from build123d import *

# Parameters (mm, degrees)
BOSS_EXTRU_1_DEPTH      = 7
CONG_1_R                = 1
COQUE1_T                = -0.3
ENL_V_MAT_EXTRU_1_REACH = 9
ESQUISSE8_R             = 4.427961532
ENL_V_MAT_EXTRU_2_REACH = 9
ESQUISSE9_W             = 4.325203416
ESQUISSE9_H             = 7.820915767
ENL_V_MAT_EXTRU_3_REACH = 9
ESQUISSE10_W            = 4.799198311
ESQUISSE10_H            = 8.413409385


with BuildPart() as part:
    # Esquisse3 → Boss.-Extru.1 (new body)
    with BuildSketch(Plane(origin=(0, 0, 0), x_dir=(1, 0, 0), z_dir=(0, 1, 0))):
        with BuildLine():
            Line((-26.504477612, 19.954228856), (25.695522388, 19.954228856))
            ThreePointArc((25.695522388, 19.954228856), (26.402629169, 19.661335637), (26.695522388, 18.954228856))
            Line((26.695522388, 18.954228856), (26.695522388, -23.245771144))
            ThreePointArc((26.695522388, -23.245771144), (26.402629169, -23.952877925), (25.695522388, -24.245771144))
            Line((25.695522388, -24.245771144), (-26.504477612, -24.245771144))
            ThreePointArc((-26.504477612, -24.245771144), (-27.211584393, -23.952877925), (-27.504477612, -23.245771144))
            Line((-27.504477612, -23.245771144), (-27.504477612, 18.954228856))
            ThreePointArc((-27.504477612, 18.954228856), (-27.211584393, 19.661335637), (-26.504477612, 19.954228856))
        make_face()
    extrude(amount=BOSS_EXTRU_1_DEPTH)

    # Congé1
    cong_1_edges = [part.edges().sort_by_distance(p)[0] for p in [
        (26.402629169, 7, -19.661335637),
        (26.695522388, 7, 2.145771144),
        (26.402629169, 7, 23.952877925),
        (-0.404477612, 7, 24.245771144),
        (-27.211584393, 7, 23.952877925),
        (-27.504477612, 7, 2.145771144),
        (-27.211584393, 7, -19.661335637),
        (-0.404477612, 7, -19.954228856),
    ]]
    fillet(cong_1_edges, radius=CONG_1_R)

    # Coque1
    coque1_openings = [part.faces().sort_by_distance(p)[0] for p in [
        (-0.404477612, 0, 2.145771144),
    ]]
    offset(amount=COQUE1_T, openings=coque1_openings, kind=Kind.INTERSECTION)

    # Esquisse8 → Enlèv. mat.-Extru.1 (cut, up to next)
    with BuildSketch(Plane(origin=(0, 7, 0), x_dir=(1, 0, 0), z_dir=(0, 1, 0)), mode=Mode.PRIVATE) as enl_v_mat_extru_1_sk1:
        with Locations((-4.865513773, -1.564595223)):
            Circle(ESQUISSE8_R)
    enl_v_mat_extru_1_tool1 = extrude(enl_v_mat_extru_1_sk1.sketch, amount=-ENL_V_MAT_EXTRU_1_REACH, mode=Mode.PRIVATE) & part.part
    add(enl_v_mat_extru_1_tool1.solids().sort_by_distance((-4.865514, 7, 1.564595))[0], mode=Mode.SUBTRACT)

    # Esquisse9 → Enlèv. mat.-Extru.2 (cut, up to next)
    with BuildSketch(Plane(origin=(0, 7, 0), x_dir=(1, 0, 0), z_dir=(0, 1, 0)), mode=Mode.PRIVATE) as enl_v_mat_extru_2_sk1:
        with Locations((-12.89117049, 11.513635006)):
            Rectangle(ESQUISSE9_W, ESQUISSE9_H)
    enl_v_mat_extru_2_tool1 = extrude(enl_v_mat_extru_2_sk1.sketch, amount=-ENL_V_MAT_EXTRU_2_REACH, mode=Mode.PRIVATE) & part.part
    add(enl_v_mat_extru_2_tool1.solids().sort_by_distance((-12.89117, 7, -11.513635))[0], mode=Mode.SUBTRACT)

    # Esquisse10 → Enlèv. mat.-Extru.3 (cut, up to next)
    with BuildSketch(Plane(origin=(0, 7, 0), x_dir=(1, 0, 0), z_dir=(0, 1, 0)), mode=Mode.PRIVATE) as enl_v_mat_extru_3_sk1:
        with Locations((21.532708754, -8.690397391)):
            Rectangle(ESQUISSE10_W, ESQUISSE10_H)
    enl_v_mat_extru_3_tool1 = extrude(enl_v_mat_extru_3_sk1.sketch, amount=-ENL_V_MAT_EXTRU_3_REACH, mode=Mode.PRIVATE) & part.part
    add(enl_v_mat_extru_3_tool1.solids().sort_by_distance((21.532709, 7, 8.690397))[0], mode=Mode.SUBTRACT)


solid = part.part
Read the model definition and answer for the solid it produces. Units are mm, in the model's axes. A direction names the side the tool comes from. Coordinates: 2 decimals unless noted, no trailing zeros. Write each loop counter-clockwise with the first axis right and the second up, starting at its lowest first coordinate (ties: lowest second). Pieces come first, ordered by that corner, then holes. Notation, with made-up numbers: M -24,40.5 L 28,40.5 A30 cw 28,78.5 Z; hole C -7,-2 d5. An arc over 180 degrees is marked long. Use a Markdown table: item, result.
Q1. Each of these flat-tipped pins is pushed along its axis until it touches: pin 1 Ø10 at (x, z) = (-4.87, 1.56) entering from +Y; pin 2 Ø3 at (x, z) = (20.5, -2) entering from -Y. Where does it stop, or does it pass through?
Answer block:
| item | result |
|---|---|
| pin 1 | stops at y = 7 |
| pin 2 | stops at y = 6.7 |
Q2. Straight lines are drawn through the part: L1, parallel to X at y = 0.5, z = -1; L2, parallel to Z at x = -17.5, y = 3.5; L3, parallel to Y at x = -15.5, z = 17. For each, find the intervals that lie inside material, in ascending order. Write a range as [from, to].
Answer block:
| item | result |
|---|---|
| L1 | x = [-27.5, -27.2], [26.4, 26.7] |
| L2 | z = [-19.95, -19.65], [23.95, 24.25] |
| L3 | y = [6.7, 7] |
Q3. Determine the mould class of faces 3 (the face through (-1, 3, -19.954)), 4 (the face through (-27.504, 3, 2)), 5 (the face through (-2.82, 6.85, 5.49)) for opening direction Z: released by +Z, released by -Z, zero draft, split by the parting line, or undercut.
Answer block:
| item | result |
|---|---|
| face 3 | released by -Z |
| face 4 | zero draft |
| face 5 | undercut |
Q4. The part is cut by section D-D, the plane z = 14. Write down the section's boundary in (x, y), then the cut area to 3 significant figures.
Answer block:
| item | result |
|---|---|
| outline | M -27.5,0 L -27.2,0 L -27.2,6 A0.7 cw -26.5,6.7 L 25.7,6.7 A0.7 cw 26.4,6 L 26.4,0 L 26.7,0 L 26.7,6 A1 ccw 25.7,7 L -26.5,7 A1 ccw -27.5,6 Z |
| area | 20.1 mm2 |
Q5. The part is cut by section C-C, the plane x = -4. Write down the section's boundary in (y, z).
Answer block:
| item | result |
|---|---|
| outline | M 0,-19.95 L 6,-19.95 A1 ccw 7,-18.95 L 7,-2.78 L 6.7,-2.78 L 6.7,-18.95 A0.7 cw 6,-19.65 L 0,-19.65 Z; M 0,23.95 L 6,23.95 A0.7 cw 6.7,23.25 L 6.7,5.91 L 7,5.91 L 7,23.25 A1 ccw 6,24.25 L 0,24.25 Z |
Q6. Which of the six approach directions +Z, -Z, +X, -X, +Y, -Y give full straight-line access (tool end or side, diameter ignored) to faces 1 (the face through (0, 7, 2)), 2 (the face through (0, 3, 23.946))?
Answer block:
| item | result |
|---|---|
| face 1 | +Z, -Z, +X, -X, +Y |
| face 2 | -Y |
Q7. The part is cut by section B-B, the plane y = 5.25. Write down the section's boundary in (x, z), then the cut area to 3 significant figures.
Answer block:
| item | result |
|---|---|
| outline | M -27.5,-18.95 A1 ccw -26.5,-19.95 L 25.7,-19.95 A1 ccw 26.7,-18.95 L 26.7,23.25 A1 ccw 25.7,24.25 L -26.5,24.25 A1 ccw -27.5,23.25 Z; hole M -27.2,-18.95 A0.7 ccw -26.5,-19.65 L 25.7,-19.65 A0.7 ccw 26.4,-18.95 L 26.4,23.25 A0.7 ccw 25.7,23.95 L -26.5,23.95 A0.7 ccw -27.2,23.25 Z |
| area | 58.2 mm2 |
Q8. The part is cut by section A-A, the plane z = -10.5. Write down the section's boundary in (x, y).
Answer block:
| item | result |
|---|---|
| outline | M -27.5,0 L -27.2,0 L -27.2,6 A0.7 cw -26.5,6.7 L -15.05,6.7 L -15.05,7 L -26.5,7 A1 ccw -27.5,6 Z; M -10.73,6.7 L 25.7,6.7 A0.7 cw 26.4,6 L 26.4,0 L 26.7,0 L 26.7,6 A1 ccw 25.7,7 L -10.73,7 Z |
